Drawing for the job (mm, zero at the part's lowest x, y, z). A direction names the side the tool comes from. Coordinates: 2 decimals unless noted, no trailing zeros. Write each loop counter-clockwise with the first axis right and the second up, starting at its lowest first coordinate (ties: lowest second). Pieces come first, ordered by that corner, then holes. Notation, with made-up numbers: M -22,63.25 L -10,63.25 A36 cw -10,99.25 Z; hole C 44,-4.5 d3. An arc over 180 degrees is marked long. Use a Markdown table: item, result. Add a question column.
Q1. Tool access for the marked faces 5, 6 and 7: list every direction of +Z, -Z, +X, -X, +Y, -Y with a clear straight run to the whole face (end or side of a thin tool).
Q2. Pin check, flat tips, straight feed: pin 1 Ø7.5 at (x, z) = (7.5, 10.5) entering from +Y; pin 2 Ø8.5 at (y, z) = (48.5, 10) entering from -X; pin 3 Ø6 at (y, z) = (48.5, 14) entering from +X. Stop position of each tip, or through.
Q3. Wall check: L1, parallel to X at y = 32, z = 12; L2, parallel to Y at x = 20.5, z = 10; L3, parallel to Y at x = 27, z = 10. Give the ranges that are in metal, low to high. Write a range as from..to.
Q4. Slice it at B-B on x = 7.5. Write the cut outline in (y, z).
Q5. Mould opens along Z. For the marked faces 1, 2, 3 and 4 say: released by +Z, released by -Z, zero draft, split by the parting line, or undercut.
Q6. Slice it at C-C on z = 16.25. Write the cut outline in (x, y).
Q7. Slice it at A-A on y = 32. Write the cut outline in (x, z), then the cut area to 3 significant figures.
Q8. Slice it at D-D on y = 9. Write the cut outline in (x, z).
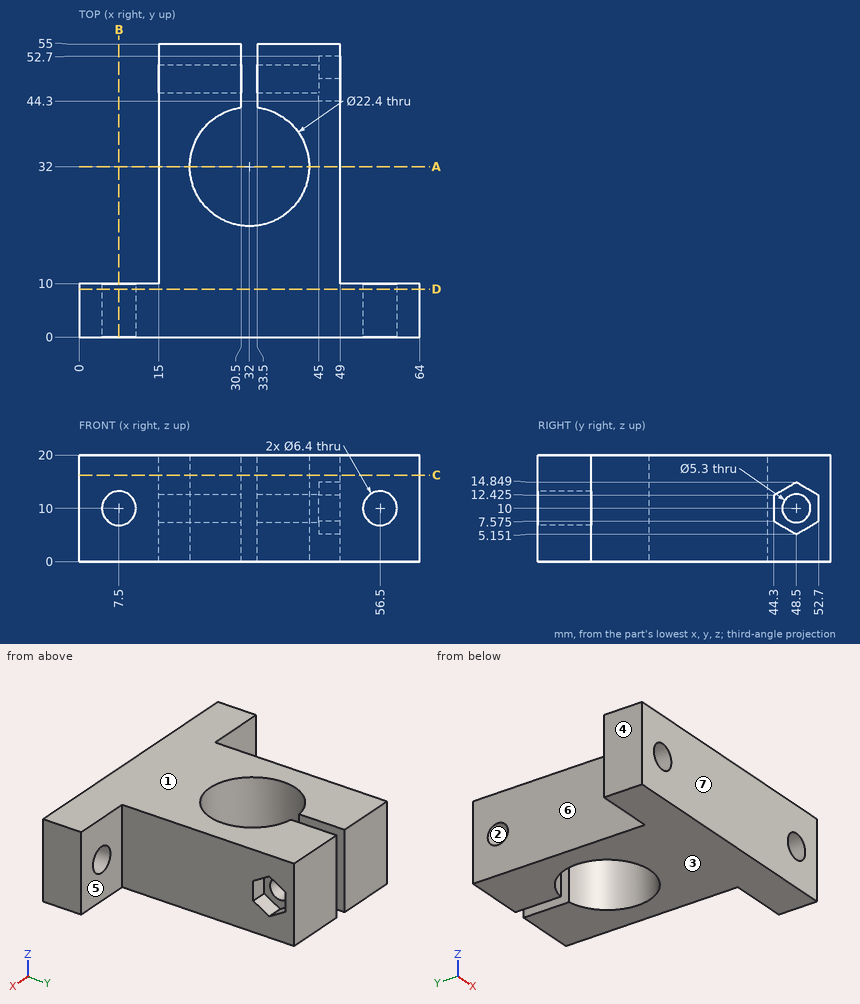
Recorded:
| question | item | result |
|---|---|---|
| 1 | face 5 | +Z, -Z, +X, +Y |
| 1 | face 6 | +Z, -Z, -X, +Y |
| 1 | face 7 | +Z, -Z, +X, -X, -Y |
| 2 | pin 1 | y = 10 |
| 2 | pin 2 | x = 15 |
| 2 | pin 3 | x = 49 |
| 3 | L1 | 15..20.8, 43.2..49 |
| 3 | L2 | 0..45.85, 51.15..55 |
| 3 | L3 | 0..21.98, 42.02..45.85, 51.15..55 |
| 4 | outline | M 0,0 L 10,0 L 10,6.8 L 0,6.8 Z; M 0,13.2 L 10,13.2 L 10,20 L 0,20 Z |
| 5 | face 1 | released by +Z |
| 5 | face 2 | undercut |
| 5 | face 3 | released by -Z |
| 5 | face 4 | zero draft |
| 6 | outline | M 0,0 L 64,0 L 64,10 L 49,10 L 49,55 L 33.5,55 L 33.5,43.1 A11.2 cw long 30.5,43.1 L 30.5,55 L 15,55 L 15,10 L 0,10 Z |
| 7 | outline | M 15,0 L 20.8,0 L 20.8,20 L 15,20 Z; M 43.2,0 L 49,0 L 49,20 L 43.2,20 Z |
| 7 | area | 232 mm² |
| 8 | outline | M 0,0 L 64,0 L 64,20 L 0,20 Z; hole C 7.5,10 d6.4; hole C 56.5,10 d6.4 |
